from build123d import *

# Parameters (mm, degrees)
SKETCH1_W           = 12.7
SKETCH1_H           = 12.7
BOSS_EXTRUDE1_DEPTH = 2.54
FILLET1_R           = 0.635
SHELL1_START        = 0.635
SHELL1_OUTLINE_W    = 1.905
SHELL1_OUTLINE_H    = 11.43
SHELL1_DEPTH        = 11.43
SKETCH2_R           = 2.54
BOSS_EXTRUDE2_DEPTH = 1.905
BOSS_EXTRUDE3_DEPTH = 0.00254


# Read off the part's stored shape, not the designer's step: Shell1
with BuildPart() as part:
    # Sketch1 → Boss-Extrude1 (new body)
    with BuildSketch(Plane(origin=(0, 0, 0), x_dir=(1, 0, 0), z_dir=(0, 1, 0))):
        with Locations((6.35, 6.35)):
            Rectangle(SKETCH1_W, SKETCH1_H)
    extrude(amount=BOSS_EXTRUDE1_DEPTH)

    # Fillet1
    fillet1_edges = [part.edges().sort_by_distance(p)[0] for p in [
        (0, 1.27, -12.7),
        (12.7, 1.27, -12.7),
        (12.7, 1.27, 0),
        (0, 1.27, 0),
    ]]
    fillet(fillet1_edges, radius=FILLET1_R)

    # Shell1 outline → Shell1 (cut)
    with BuildSketch(Plane.YZ.offset(SHELL1_START)):
        with Locations((0.9525, -6.35)):
            Rectangle(SHELL1_OUTLINE_W, SHELL1_OUTLINE_H)
    extrude(amount=SHELL1_DEPTH, mode=Mode.SUBTRACT)

    # Sketch2 → Boss-Extrude2 (add)
    with BuildSketch(Plane(origin=(0, 1.905, 0), x_dir=(-1, 0, 0), z_dir=(0, -1, 0))):
        with Locations(Location((-6.35, 6.35, 0), (0, 0, 270))):
            Circle(SKETCH2_R)
    extrude(amount=BOSS_EXTRUDE2_DEPTH)

    # Sketch3 → Boss-Extrude3 (add)
    with BuildSketch(Plane(origin=(0, 2.54, 0), x_dir=(1, 0, 0), z_dir=(0, 1, 0))):
        with BuildLine():
            Line((5.192346154, 8.001), (5.856348558, 8.001))
            add(Edge.make_bspline(
                [(5.856348558, 8.001), (5.900238914, 8.000844214), (5.984652434, 8.000544595), (6.106372118, 7.995817392), (6.218188387, 7.989239101), (6.320266796, 7.979200455), (6.412563672, 7.965890424), (6.49517152, 7.950200099), (6.568087924, 7.93231761), (6.631927834, 7.910034619), (6.689540196, 7.884899742), (6.743242928, 7.856019307), (6.79422079, 7.823714908), (6.842133051, 7.787136528), (6.887396081, 7.746942202), (6.93009527, 7.703091473), (6.969627239, 7.655212502), (7.005747205, 7.603607826), (7.038667646, 7.54932089), (7.067762412, 7.492277157), (7.091422324, 7.432436959), (7.112328392, 7.370665114), (7.127386356, 7.306078583), (7.13785895, 7.239306125), (7.145526573, 7.170112696), (7.145967424, 7.123105753), (7.146192308, 7.099127003)],
                knots=[0, 0, 0, 0, 1.749336639, 3.364467119, 4.854658419, 6.213483162, 7.451590619, 8.570285859, 9.5643256, 10.440900261, 11.26203566, 12.067320669, 12.869050712, 13.665104639, 14.467235401, 15.27997916, 16.102287765, 16.939272006, 17.78853747, 18.631303466, 19.488103222, 20.351255419, 21.228522269, 22.127379805, 23.044756219, 24, 24, 24, 24], degree=3))
            add(Edge.make_bspline(
                [(7.146192308, 7.099127003), (7.145608142, 7.074098697), (7.1444627, 7.025022751), (7.138292723, 6.952934188), (7.127015945, 6.883964894), (7.109935624, 6.818316801), (7.090304013, 6.755172843), (7.064199007, 6.695698066), (7.034736927, 6.639027495), (6.999745675, 6.585962756), (6.961344486, 6.535325176), (6.916684711, 6.489054868), (6.868659617, 6.444664978), (6.814569539, 6.404935939), (6.756798818, 6.367181417), (6.694199611, 6.332965765), (6.627180461, 6.301428881), (6.580062679, 6.283841737), (6.555967949, 6.274848157)],
                knots=[0, 0, 0, 0, 1.099860209, 2.156625411, 3.176576793, 4.16617041, 5.135385252, 6.078461593, 7.016046972, 7.938469504, 8.868247731, 9.803980173, 10.76021508, 11.73834243, 12.748633912, 13.790971185, 14.870363756, 16, 16, 16, 16], degree=3))
            Line((6.555967949, 6.274848157), (7.288660256, 4.826))
            Line((7.288660256, 4.826), (6.655186699, 4.826))
            Line((6.655186699, 4.826), (5.955567308, 6.209974359))
            Line((5.955567308, 6.209974359), (5.762217949, 6.209974359))
            Line((5.762217949, 6.209974359), (5.762217949, 4.826))
            Line((5.762217949, 4.826), (5.192346154, 4.826))
            Line((5.192346154, 4.826), (5.192346154, 8.001))
        make_face()
        with BuildLine():
            Line((5.762217949, 6.779846154), (5.984188101, 6.779846154))
            add(Edge.make_bspline(
                [(5.984188101, 6.779846154), (6.011325797, 6.780151797), (6.063288654, 6.780737037), (6.138018068, 6.783451626), (6.205890197, 6.789992443), (6.267196508, 6.798256521), (6.322245489, 6.807798593), (6.370546122, 6.82147296), (6.412842646, 6.836125392), (6.448633846, 6.854334563), (6.479213025, 6.87504234), (6.505616188, 6.898566889), (6.52745539, 6.92579356), (6.545430168, 6.955982448), (6.55941259, 6.989400567), (6.569618687, 7.025681062), (6.575322386, 7.065237214), (6.575978616, 7.092536345), (6.576320513, 7.106759215)],
                knots=[0, 0, 0, 0, 1.688639943, 3.233382647, 4.650958383, 5.928841754, 7.082724185, 8.122798841, 9.049171256, 9.863274652, 10.613301712, 11.341792392, 12.054588806, 12.776240173, 13.521029143, 14.301969904, 15.115324896, 16, 16, 16, 16], degree=3))
            add(Edge.make_bspline(
                [(6.576320513, 7.106759215), (6.575674126, 7.123585908), (6.57440442, 7.15663883), (6.561804988, 7.204223447), (6.541749414, 7.248266266), (6.514258716, 7.28856829), (6.479637754, 7.323899827), (6.43990747, 7.355044858), (6.394210387, 7.379672018), (6.351898327, 7.39591583), (6.313404242, 7.405634671), (6.278664546, 7.412877065), (6.238435767, 7.418009958), (6.192687537, 7.423454304), (6.14153647, 7.426984687), (6.08470376, 7.429561163), (6.022352631, 7.430615326), (5.978887972, 7.430952323), (5.956203325, 7.431128205)],
                knots=[0, 0, 0, 0, 1.020303359, 2.004196876, 2.966617323, 3.9489082, 4.950758222, 5.960522915, 7.003732012, 8.091992268, 8.70421221, 9.413913587, 10.24622431, 11.166358409, 12.212345909, 13.359657661, 14.621978493, 16, 16, 16, 16], degree=3))
            Line((5.956203325, 7.431128205), (5.762217949, 7.431128205))
            Line((5.762217949, 7.431128205), (5.762217949, 6.779846154))
        make_face(mode=Mode.SUBTRACT)
    extrude(amount=BOSS_EXTRUDE3_DEPTH)


solid = part.part
Verification items for the finished model (mm, model axes). A direction names the side the tool comes from. Give positions to 0.01 mm unless a question says otherwise; leave off trailing zeros. Write each loop counter-clockwise with the first axis right and the second up, starting at its lowest first coordinate (ties: lowest second). Pieces come first, ordered by that corner, then holes.
(1) Gauge pin test, flat end, axial feed: pin 1 (4 mm diameter, centred on x = 3.5, z = -4, fed in from +Y). Record the tip position at first contact, or that the pin passes through.
(2) Cross-section at A-A (y = 1.25). Enter the section's corners in (x, z) (3 decimals).
(3) Material ranges on line 1 (Z direction, x = 11, y = 0.35) (3 decimals); line 2 (X direction, y = 1.7, z = -6.25) (3 decimals); line 3 (Z direction, x = 5, y = 1.1) (3 decimals), recorded low to high.
(4) Access from +Z, -Z, +X, -X, +Y, -Y to the whole of each face (thin tool, end or side, straight path). Record for faces 1 (the face through (6, 1, -0.635)), 2 (the face through (6, 2.543, -6.4)).
(5) Cross-section at B-B (x = 1.5). Enter the section's corners in (y, z) (3 decimals), plus the area to 3 significant figures.
(6) Cross-section at C-C (z = -2.5). Enter the section's corners in (x, y) (3 decimals).
(7) Mould release check, pull along Z, two halves, no side actions. Record for faces 3 (the face through (6, 1, -12.7)), 4 (the face through (12.065, 1, -6)), 5 (the face through (12.7, 1, -6)): +Z half, -Z half, draft (parallel to the pull), parting line (faces both ways), or undercut.
Worked out:
1. pin 1: stops at y = 2.54
2. outline: (0, -12.065) arc R0.635 ccw to (0.635, -12.7) - (12.065, -12.7) arc R0.635 ccw to (12.7, -12.065) - (12.7, -0.635) arc R0.635 ccw to (12.065, 0) - (0.635, 0) arc R0.635 ccw to (0, -0.635) - close; circle Ø5.08 at (6.35, -6.35); hole (0.635, -12.065) - (12.065, -12.065) - (12.065, -0.635) - (0.635, -0.635) - close
3. line 1: z = -12.7 to -12.065, -0.635 to 0
3. line 2: x = 0 to 0.635, 3.812 to 8.888, 12.065 to 12.7
3. line 3: z = -12.7 to -12.065, -8.502 to -4.198, -0.635 to 0
4. face 1: -Y
4. face 2: +Z, -Z, +X, -X, +Y
5. outline: (0, -12.7) - (2.54, -12.7) - (2.54, 0) - (0, 0) - (0, -0.635) - (1.905, -0.635) - (1.905, -12.065) - (0, -12.065) - close
5. area: 10.5 mm2
6. outline: (0, 0) - (0.635, 0) - (0.635, 1.905) - (12.065, 1.905) - (12.065, 0) - (12.7, 0) - (12.7, 2.54) - (0, 2.54) - close
7. face 3: -Z half
7. face 4: undercut
7. face 5: draft
